from build123d import *

# Parameters (mm, degrees)
F0_R         = 55
F0_R_2       = 1
F0_R_3       = 2.5
F0_R_4       = 10
F1_DEPTH     = 50
F1_FACE_R    = 55
F1_FACE_R_2  = 1
F1_FACE_R_3  = 2.5
F2_DEPTH     = 40
F3_R         = 7.5
F3_R_2       = 2.5
F4_DEPTH     = 5
F6_DEPTH     = 25
F7_DEPTH     = 5
F8_T4_DEPTH  = 15.1824583655
F8_S5_R      = 10
F8_T6_DEPTH  = 9
F8_T10_DEPTH = 15.1824583655
F8_S11_R     = 10
F8_T12_DEPTH = 9
F8_T16_DEPTH = 15.1824583655
F8_S17_R     = 10
F8_T18_DEPTH = 9
F8_T22_DEPTH = 15.1824583655
F8_S23_R     = 10
F8_T24_DEPTH = 9


# Not quite as in the source:
# - a fillet or chamfer that OpenCascade refuses, or shapes differently, is made with other operations: its cross-section is extruded or revolved along the edge and cut away or added


with BuildPart() as f1:
    # F0 (on Top) → F1 (new body)
    with BuildSketch(Plane.XY):
        Circle(F0_R)
        with Locations((-26, -45.0333209968)):
            Circle(F0_R_2, mode=Mode.SUBTRACT)
        with Locations((-48.8640162809, -17.7850474529)):
            Circle(F0_R_2, mode=Mode.SUBTRACT)
        with Locations((-15, -25.9807621135)):
            Circle(F0_R_3, mode=Mode.SUBTRACT)
        with Locations((9.0297052387, -51.2100031566)):
            Circle(F0_R_2, mode=Mode.SUBTRACT)
        with Locations((39.8343110422, -33.4249557037)):
            Circle(F0_R_2, mode=Mode.SUBTRACT)
        with Locations((15, -25.9807621135)):
            Circle(F0_R_3, mode=Mode.SUBTRACT)
        with Locations((-30, 0)):
            Circle(F0_R_3, mode=Mode.SUBTRACT)
        with Locations((-48.8640162809, 17.7850474529)):
            Circle(F0_R_2, mode=Mode.SUBTRACT)
        with Locations((-15, 25.9807621135)):
            Circle(F0_R_3, mode=Mode.SUBTRACT)
        with Locations((-26, 45.0333209968)):
            Circle(F0_R_2, mode=Mode.SUBTRACT)
        Circle(F0_R_4, mode=Mode.SUBTRACT)
        with Locations((15, 25.9807621135)):
            Circle(F0_R_3, mode=Mode.SUBTRACT)
        with Locations((30, 0)):
            Circle(F0_R_3, mode=Mode.SUBTRACT)
        with Locations((52, 0)):
            Circle(F0_R_2, mode=Mode.SUBTRACT)
        with Locations((9.0297052387, 51.2100031566)):
            Circle(F0_R_2, mode=Mode.SUBTRACT)
        with Locations((39.8343110422, 33.4249557037)):
            Circle(F0_R_2, mode=Mode.SUBTRACT)
        Circle(F0_R_4)
    extrude(amount=F1_DEPTH)

    # F0 (on Top) + F1_face (on face) → F2 (cut)
    with BuildSketch(Plane.XY):
        Circle(F0_R)
        with Locations((-26, -45.0333209968)):
            Circle(F0_R_2, mode=Mode.SUBTRACT)
        with Locations((-48.8640162809, -17.7850474529)):
            Circle(F0_R_2, mode=Mode.SUBTRACT)
        with Locations((-15, -25.9807621135)):
            Circle(F0_R_3, mode=Mode.SUBTRACT)
        with Locations((9.0297052387, -51.2100031566)):
            Circle(F0_R_2, mode=Mode.SUBTRACT)
        with Locations((39.8343110422, -33.4249557037)):
            Circle(F0_R_2, mode=Mode.SUBTRACT)
        with Locations((15, -25.9807621135)):
            Circle(F0_R_3, mode=Mode.SUBTRACT)
        with Locations((-30, 0)):
            Circle(F0_R_3, mode=Mode.SUBTRACT)
        with Locations((-48.8640162809, 17.7850474529)):
            Circle(F0_R_2, mode=Mode.SUBTRACT)
        with Locations((-15, 25.9807621135)):
            Circle(F0_R_3, mode=Mode.SUBTRACT)
        with Locations((-26, 45.0333209968)):
            Circle(F0_R_2, mode=Mode.SUBTRACT)
        Circle(F0_R_4, mode=Mode.SUBTRACT)
        with Locations((15, 25.9807621135)):
            Circle(F0_R_3, mode=Mode.SUBTRACT)
        with Locations((30, 0)):
            Circle(F0_R_3, mode=Mode.SUBTRACT)
        with Locations((52, 0)):
            Circle(F0_R_2, mode=Mode.SUBTRACT)
        with Locations((9.0297052387, 51.2100031566)):
            Circle(F0_R_2, mode=Mode.SUBTRACT)
        with Locations((39.8343110422, 33.4249557037)):
            Circle(F0_R_2, mode=Mode.SUBTRACT)
    with BuildSketch(Plane.XY.offset(50)):
        Circle(F1_FACE_R)
        with Locations((-26, -45.0333209968)):
            Circle(F1_FACE_R_2, mode=Mode.SUBTRACT)
        with Locations((-48.8640162809, -17.7850474529)):
            Circle(F1_FACE_R_2, mode=Mode.SUBTRACT)
        with Locations((-15, -25.9807621135)):
            Circle(F1_FACE_R_3, mode=Mode.SUBTRACT)
        with Locations((9.0297052387, -51.2100031566)):
            Circle(F1_FACE_R_2, mode=Mode.SUBTRACT)
        with Locations((39.8343110422, -33.4249557037)):
            Circle(F1_FACE_R_2, mode=Mode.SUBTRACT)
        with Locations((15, -25.9807621135)):
            Circle(F1_FACE_R_3, mode=Mode.SUBTRACT)
        with Locations((-30, 0)):
            Circle(F1_FACE_R_3, mode=Mode.SUBTRACT)
        with Locations((-48.8640162809, 17.7850474529)):
            Circle(F1_FACE_R_2, mode=Mode.SUBTRACT)
        with Locations((-15, 25.9807621135)):
            Circle(F1_FACE_R_3, mode=Mode.SUBTRACT)
        with Locations((-26, 45.0333209968)):
            Circle(F1_FACE_R_2, mode=Mode.SUBTRACT)
        with Locations((15, 25.9807621135)):
            Circle(F1_FACE_R_3, mode=Mode.SUBTRACT)
        with Locations((30, 0)):
            Circle(F1_FACE_R_3, mode=Mode.SUBTRACT)
        with Locations((52, 0)):
            Circle(F1_FACE_R_2, mode=Mode.SUBTRACT)
        with Locations((9.0297052387, 51.2100031566)):
            Circle(F1_FACE_R_2, mode=Mode.SUBTRACT)
        with Locations((39.8343110422, 33.4249557037)):
            Circle(F1_FACE_R_2, mode=Mode.SUBTRACT)
    extrude(amount=F2_DEPTH, mode=Mode.SUBTRACT)

    # F3 (on face) → F4 (cut)
    with BuildSketch(Plane(origin=(0, 0, 40), x_dir=(1, 0, 0), z_dir=(0, 0, -1))):
        with Locations((15, -25.9807621135)):
            Circle(F3_R)
        with Locations((15, -25.9807621135)):
            Circle(F3_R_2, mode=Mode.SUBTRACT)
        with Locations((30, 0)):
            Circle(F3_R)
        with Locations((30, 0)):
            Circle(F3_R_2, mode=Mode.SUBTRACT)
        with Locations((-15, -25.9807621135)):
            Circle(F3_R)
        with Locations((-15, -25.9807621135)):
            Circle(F3_R_2, mode=Mode.SUBTRACT)
        with Locations((15, 25.9807621135)):
            Circle(F3_R)
        with Locations((15, 25.9807621135)):
            Circle(F3_R_2, mode=Mode.SUBTRACT)
        with Locations((-15, 25.9807621135)):
            Circle(F3_R)
        with Locations((-15, 25.9807621135)):
            Circle(F3_R_2, mode=Mode.SUBTRACT)
        with Locations((-30, 0)):
            Circle(F3_R)
        with Locations((-30, 0)):
            Circle(F3_R_2, mode=Mode.SUBTRACT)
    extrude(amount=-F4_DEPTH, mode=Mode.SUBTRACT)

    # F5 (on face) → F6 (cut)
    with BuildSketch(Plane(origin=(0, 0, 0), x_dir=(1, 0, 0), z_dir=(0, 0, -1))):
        with BuildLine():
            Line((-2.5, 7), (0, 7))
            Line((0, 7), (2.5, 7))
            Line((2.5, 7), (2.5, 9.6824583655))
            ThreePointArc((2.5, 9.6824583655), (0, 10), (-2.5, 9.6824583655))
            Line((-2.5, 9.6824583655), (-2.5, 7))
        make_face()
    extrude(amount=-F6_DEPTH, mode=Mode.SUBTRACT)

    # F5 (on face) → F7 (join)
    with BuildSketch(Plane(origin=(0, 0, 0), x_dir=(1, 0, 0), z_dir=(0, 0, -1))):
        with BuildLine():
            Line((-2.5, 7), (0, 7))
            Line((0, 7), (2.5, 7))
            Line((2.5, 7), (2.5, 9.6824583655))
            ThreePointArc((2.5, 9.6824583655), (0, 10), (-2.5, 9.6824583655))
            Line((-2.5, 9.6824583655), (-2.5, 7))
        make_face()
    extrude(amount=-F7_DEPTH)

    # F8: fillet of radius 2.5 on 4 edges, made by hand


with BuildPart() as f8_tool2:
    # F8_s3 → F8_t4 (new body)
    with BuildSketch(Plane.XZ.offset(15.9324583655)):
        with BuildLine():
            ThreePointArc((-2.5, 22.5), (-1.767766953, 24.267766953), (0, 25))
            Line((0, 25), (-2.5, 25))
            Line((-2.5, 25), (-2.5, 22.5))
        make_face()
    extrude(amount=-F8_T4_DEPTH)

    # F8_s5 → F8_t6 (intersect, symmetric)
    with BuildSketch(Plane.XY.offset(23.8)):
        Circle(F8_S5_R)
    extrude(amount=F8_T6_DEPTH, both=True, mode=Mode.INTERSECT)


with BuildPart() as f1_1:
    add(f1.part)

    # F8_t1: union F8_tool2
    add(f8_tool2.part)


with BuildPart() as f8_tool8:
    # F8_s9 → F8_t10 (new body)
    with BuildSketch(Plane.XZ.offset(0.75)):
        with BuildLine():
            ThreePointArc((0, 25), (1.767766953, 24.267766953), (2.5, 22.5))
            Line((2.5, 22.5), (2.5, 25))
            Line((2.5, 25), (0, 25))
        make_face()
    extrude(amount=F8_T10_DEPTH)

    # F8_s11 → F8_t12 (intersect, symmetric)
    with BuildSketch(Plane.XY.offset(23.8)):
        Circle(F8_S11_R)
    extrude(amount=F8_T12_DEPTH, both=True, mode=Mode.INTERSECT)


with BuildPart() as f1_2:
    add(f1_1.part)

    # F8_t7: union F8_tool8
    add(f8_tool8.part)


with BuildPart() as f8_tool14:
    # F8_s15 → F8_t16 (new body)
    with BuildSketch(Plane.XZ.offset(0.75)):
        with BuildLine():
            ThreePointArc((2.5, 7.5), (1.767766953, 5.732233047), (0, 5))
            Line((0, 5), (2.5, 5))
            Line((2.5, 5), (2.5, 7.5))
        make_face()
    extrude(amount=F8_T16_DEPTH)

    # F8_s17 → F8_t18 (intersect, symmetric)
    with BuildSketch(Plane.XY.offset(6.2)):
        Circle(F8_S17_R)
    extrude(amount=F8_T18_DEPTH, both=True, mode=Mode.INTERSECT)


with BuildPart() as f1_3:
    add(f1_2.part)

    # F8_t13: union F8_tool14
    add(f8_tool14.part)


with BuildPart() as f8_tool20:
    # F8_s21 → F8_t22 (new body)
    with BuildSketch(Plane.XZ.offset(15.9324583655)):
        with BuildLine():
            ThreePointArc((-2.5, 7.5), (-1.767766953, 5.732233047), (0, 5))
            Line((0, 5), (-2.5, 5))
            Line((-2.5, 5), (-2.5, 7.5))
        make_face()
    extrude(amount=-F8_T22_DEPTH)

    # F8_s23 → F8_t24 (intersect, symmetric)
    with BuildSketch(Plane.XY.offset(6.2)):
        Circle(F8_S23_R)
    extrude(amount=F8_T24_DEPTH, both=True, mode=Mode.INTERSECT)


with BuildPart() as f1_4:
    add(f1_3.part)

    # F8_t19: union F8_tool20
    add(f8_tool20.part)


solid = f1_4.part
Geometry: final body of the model. Coordinates: model frame, mm. A direction names the side the tool comes from. Coordinates: 2 decimals unless noted, no trailing zeros. Write each loop counter-clockwise with the first axis right and the second up, starting at its lowest first coordinate (ties: lowest second). Pieces come first, ordered by that corner, then holes. Notation, with made-up numbers: (66.25, 36) - (119.25, 36) arc R29 ccw to (119.25, 59) - close; hole circle Ø10 at (40.25, 70.25). An arc over 180 degrees is marked (long way). Return JSON: item names as keys, results as strings.
Item 1: Line query: L1, parallel to Y at x = -26, z = 44.5; L2, parallel to Y at x = 15, z = 46.85; L3, parallel to Y at x = -21.5, z = 40.5. Output: solid intervals per line, ascending.
Completed:
{"L1": "y = -48.47 to -46.03, -44.03 to -6.34, 6.34 to 44.03, 46.03 to 48.47", "L2": "y = -52.92 to -28.48, -23.48 to 23.48, 28.48 to 52.92", "L3": "y = -50.62 to -29.72, -22.24 to 22.24, 29.72 to 50.62"}
Item 2: Reachability of faces 1 (the face through (13.37, -18.66, 42.46)), 2 (the face through (-32.5, 0.1, 47.5)), 3 (the face through (2.5, -8, 15)) from +Z, -Z, +X, -X, +Y, -Y: full face, straight path, thin tool, end or side. Return the list, or none.
Completed:
{"face 1": "-Z", "face 2": "+Z, -Z", "face 3": "-Y"}
Item 3: Section query D-D (y = 42). Output: boundary loops of the cut face in (x, z).
Completed:
{"outline": "(-35.51, 40) - (35.51, 40) - (35.51, 50) - (-35.51, 50) - close"}
Item 4: Section query C-C (y = 20.5). Output: boundary loops of the cut face in (x, z).
Completed:
{"outline": "(-51.04, 40) - (-20.12, 40) - (-20.12, 45) - (-9.88, 45) - (-9.88, 40) - (9.88, 40) - (9.88, 45) - (20.12, 45) - (20.12, 40) - (51.04, 40) - (51.04, 50) - (-51.04, 50) - close"}
Item 5: Pull-direction query (Y, two-part tool) for faces 4 (the face through (-11.923, -53.692, 44.93)), 5 (the face through (13.157, 27.67, 47.465)), 6 (the face through (-2.5, -8, 15)); classes: +Y half, -Y half, draft (parallel to the pull), parting line (faces both ways), or undercut.
Completed:
{"face 4": "parting line", "face 5": "undercut", "face 6": "draft"}
Item 6: Pin query (flat end, axial travel): pin 1 Ø12 at (x, y) = (18.5, 24) entering from -Z; pin 2 Ø1.5 at (x, z) = (-0.5, 11.5) entering from -Y; pin 3 Ø3 at (x, z) = (-9.5, 32.5) entering from -Y. Return the tip coordinate at first contact, or that it passes through.
Completed:
{"pin 1": "stops at z = 40", "pin 2": "stops at y = -7", "pin 3": "stops at y = -6"}
Item 7: Section query B-B (z = 42.5). Count the separate pieces of the cut face and the enclosed holes in it, and give its area (3 significant figures).
Completed:
{"separate pieces": "1", "enclosed holes": "15", "area": "8,410 mm2"}
Item 8: Section query A-A (x = 14.5). Output: boundary loops of the cut face in (y, z), and give its area (3 significant figures).
Completed:
{"outline": "(-53.05, 40) - (-33.46, 40) - (-33.46, 45) - (-28.43, 45) - (-28.43, 50) - (-53.05, 50) - close; (-23.53, 45) - (-18.5, 45) - (-18.5, 40) - (18.5, 40) - (18.5, 45) - (23.53, 45) - (23.53, 50) - (-23.53, 50) - close; (28.43, 45) - (33.46, 45) - (33.46, 40) - (53.05, 40) - (53.05, 50) - (28.43, 50) - close", "area": "862 mm2"}
